For this review, take the finished solid that the model builds, in its own axes (mm). Coordinates: 2 decimals unless noted, no trailing zeros. Write each loop counter-clockwise with the first axis right and the second up, starting at its lowest first coordinate (ties: lowest second). Pieces come first, ordered by that corner, then holes.
1) We need section D-D on y = -16.5. Give the number of separate pieces and of enclosed holes in the cut face, then the cut area to 3 significant figures.
2) We need section C-C on z = -9. Write out the cut boundary in (x, y).
3) We need section B-B on z = 36. Write out the cut boundary in (x, y), then the cut area to 3 significant figures.
4) Insertion check: P1, Ø14.5, axis at x = 15, z = -41.11, coming from the +Y side. The pin has a flat end and moves straight along its axis. Give the tip position at first contact, or say it passes through.
5) To check wall thickness, follow line 1 along X through (y, z) = (-7.5, -72.5); line 2 along X through (y, z) = (-2.25, 85); line 3 along X through (y, z) = (-7.75, 78.5). State the ranges of each line that lie inside material, in increasing order.
6) We need section A-A on z = -41.11. Write out the cut boundary in (x, y), then the cut area to 3 significant figures.
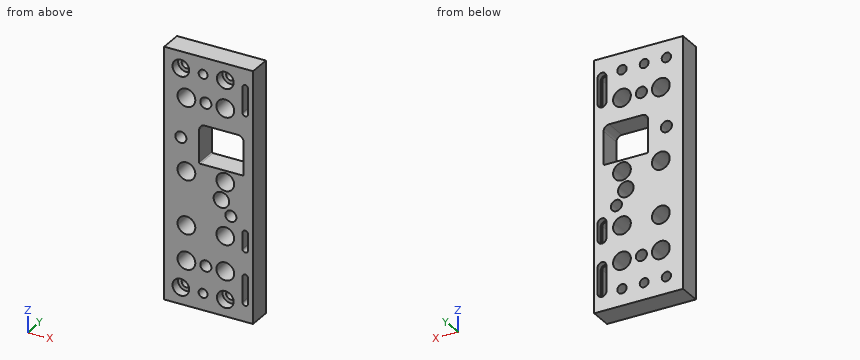
from build123d import *

# Parameters (mm, degrees)
SKETCH1_W                                    = 80
SKETCH1_H                                    = 225
BOSS_EXTRUDE1_DEPTH                          = 20
CUT_EXTRUDE1_REACH                           = 123.063
CUT_EXTRUDE2_REACH                           = 123.063
CUT_EXTRUDE3_DEPTH                           = 5
CBORE_FOR_M8_HEX_SOCKET_HEAD_CAP_SCR_2_COUNT = 2
CBORE_FOR_M8_HEX_SOCKET_HEAD_CAP_SCR_2_PITCH = 40
CBORE_FOR_M8_HEX_SOCKET_HEAD_CAP_SCR_3_COUNT = 2
CBORE_FOR_M8_HEX_SOCKET_HEAD_CAP_SCR_3_PITCH = 199.060292374
CBORE_FOR_M8_HEX_SOCKET_HEAD_CAP_SCR_4_COUNT = 2
CBORE_FOR_M8_HEX_SOCKET_HEAD_CAP_SCR_4_PITCH = 195
F_8_0MM_DOWEL_HOLE1_D                        = 8
F_8_0MM_DOWEL_HOLE1_CSINK_D                  = 8.05
F_8_0MM_DOWEL_HOLE1_CSINK_ANGLE              = 90
CUT_EXTRUDE4_REACH                           = 123.063
SKETCH13_R                                   = 8
CUT_EXTRUDE5_REACH                           = 123.063
SKETCH15_R                                   = 5
CUT_EXTRUDE6_REACH                           = 123.063
SKETCH17_R                                   = 7


with BuildPart() as part:
    # Sketch1 → Boss-Extrude1 (new body)
    with BuildSketch(Plane(origin=(0, 0, 0), x_dir=(1, 0, 0), z_dir=(0, 1, 0))):
        Rectangle(SKETCH1_W, SKETCH1_H)
    extrude(amount=-BOSS_EXTRUDE1_DEPTH)

    # Sketch2 → Cut-Extrude1 (cut, up to next)
    with BuildSketch(Plane(origin=(0, 0, 0), x_dir=(1, 0, 0), z_dir=(0, 1, 0)), mode=Mode.PRIVATE) as cut_extrude1_sk1:
        with BuildLine():
            Line((31.5, -47.14), (31.5, -18.14))
            ThreePointArc((31.5, -18.14), (31.207106781, -17.432893219), (30.5, -17.14))
            Line((30.5, -17.14), (-7.5, -17.14))
            ThreePointArc((-7.5, -17.14), (-8.207106781, -17.432893219), (-8.5, -18.14))
            Line((-8.5, -18.14), (-8.5, -47.14))
            ThreePointArc((-8.5, -47.14), (-7.035533906, -50.675533906), (-3.5, -52.14))
            Line((-3.5, -52.14), (26.5, -52.14))
            ThreePointArc((26.5, -52.14), (30.035533906, -50.675533906), (31.5, -47.14))
        make_face()
    cut_extrude1_tool1 = extrude(cut_extrude1_sk1.sketch, amount=-CUT_EXTRUDE1_REACH, mode=Mode.PRIVATE) & part.part
    add(cut_extrude1_tool1.solids().sort_by_distance((11.5, 0, 34.518764))[0], mode=Mode.SUBTRACT)

    # Sketch3 → Cut-Extrude2 (cut, up to next)
    with BuildSketch(Plane(origin=(0, 0, 0), x_dir=(1, 0, 0), z_dir=(0, 1, 0)), mode=Mode.PRIVATE) as cut_extrude2_sk1:
        with BuildLine():
            Line((35.5, -95.77), (35.5, -72.87))
            ThreePointArc((35.5, -72.87), (33, -70.37), (30.5, -72.87))
            Line((30.5, -72.87), (30.5, -95.77))
            ThreePointArc((30.5, -95.77), (33, -98.27), (35.5, -95.77))
        make_face()
    cut_extrude2_tool1 = extrude(cut_extrude2_sk1.sketch, amount=-CUT_EXTRUDE2_REACH, mode=Mode.PRIVATE) & part.part
    # Sketch3 → Cut-Extrude2 (cut, up to next)
    with BuildSketch(Plane(origin=(0, 0, 0), x_dir=(1, 0, 0), z_dir=(0, 1, 0)), mode=Mode.PRIVATE) as cut_extrude2_sk2:
        with BuildLine():
            Line((35.5, 33.86), (35.5, 48.36))
            ThreePointArc((35.5, 48.36), (33, 50.86), (30.5, 48.36))
            Line((30.5, 48.36), (30.5, 33.86))
            ThreePointArc((30.5, 33.86), (33, 31.36), (35.5, 33.86))
        make_face()
    cut_extrude2_tool2 = extrude(cut_extrude2_sk2.sketch, amount=-CUT_EXTRUDE2_REACH, mode=Mode.PRIVATE) & part.part
    # Sketch3 → Cut-Extrude2 (cut, up to next)
    with BuildSketch(Plane(origin=(0, 0, 0), x_dir=(1, 0, 0), z_dir=(0, 1, 0)), mode=Mode.PRIVATE) as cut_extrude2_sk3:
        with BuildLine():
            Line((35.5, 72.87), (35.5, 95.77))
            ThreePointArc((35.5, 95.77), (33, 98.27), (30.5, 95.77))
            Line((30.5, 95.77), (30.5, 72.87))
            ThreePointArc((30.5, 72.87), (33, 70.37), (35.5, 72.87))
        make_face()
    cut_extrude2_tool3 = extrude(cut_extrude2_sk3.sketch, amount=-CUT_EXTRUDE2_REACH, mode=Mode.PRIVATE) & part.part
    add(cut_extrude2_tool1.solids().sort_by_distance((33, 0, 84.32))[0], mode=Mode.SUBTRACT)
    add(cut_extrude2_tool2.solids().sort_by_distance((33, 0, -41.11))[0], mode=Mode.SUBTRACT)
    add(cut_extrude2_tool3.solids().sort_by_distance((33, 0, -84.32))[0], mode=Mode.SUBTRACT)

    # Sketch4 → Cut-Extrude3 (cut)
    with BuildSketch(Plane(origin=(0, 0, 0), x_dir=(1, 0, 0), z_dir=(0, 1, 0))):
        with BuildLine():
            Line((37, 72.87), (37, 95.77))
            ThreePointArc((37, 95.77), (33, 99.77), (29, 95.77))
            Line((29, 95.77), (29, 72.87))
            ThreePointArc((29, 72.87), (33, 68.87), (37, 72.87))
        make_face()
        with BuildLine():
            Line((37, 33.86), (37, 48.36))
            ThreePointArc((37, 48.36), (33, 52.36), (29, 48.36))
            Line((29, 48.36), (29, 33.86))
            ThreePointArc((29, 33.86), (33, 29.86), (37, 33.86))
        make_face()
        with BuildLine():
            Line((37, -95.77), (37, -72.87))
            ThreePointArc((37, -72.87), (33, -68.87), (29, -72.87))
            Line((29, -72.87), (29, -95.77))
            ThreePointArc((29, -95.77), (33, -99.77), (37, -95.77))
        make_face()
    extrude(amount=-CUT_EXTRUDE3_DEPTH, mode=Mode.SUBTRACT)

    # Sketch8 → CBORE for M8 Hex Socket Head Cap Screw1 (revolve, cut)
    with BuildSketch(Plane(origin=(-25, -20, -97.5), x_dir=(0, 0, -1), z_dir=(1, 0, 0))):
        Polygon((0, 0), (0, 20), (4.2, 20), (4.2, 8.6), (7.5, 8.6), (7.5, 0.025), (7.525, 0), align=None)
    cbore_for_m8_hex_socket_head_cap_screw1 = revolve(axis=Axis((-25, -26.35, -97.5), (0, 1, 0)), mode=Mode.SUBTRACT)

    # CBORE for M8 Hex Socket Head Cap Scr 2: CBORE for M8 Hex Socket Head Cap Screw1 ×2
    with Locations(*[(i * CBORE_FOR_M8_HEX_SOCKET_HEAD_CAP_SCR_2_PITCH, 0, 0) for i in range(1, CBORE_FOR_M8_HEX_SOCKET_HEAD_CAP_SCR_2_COUNT)]):
        add(cbore_for_m8_hex_socket_head_cap_screw1, mode=Mode.SUBTRACT)

    # CBORE for M8 Hex Socket Head Cap Scr 3: CBORE for M8 Hex Socket Head Cap Screw1 ×2
    with Locations(*[Vector(0.2009441437213313, 0, 0.9796027006414901) * (i * CBORE_FOR_M8_HEX_SOCKET_HEAD_CAP_SCR_3_PITCH) for i in range(1, CBORE_FOR_M8_HEX_SOCKET_HEAD_CAP_SCR_3_COUNT)]):
        add(cbore_for_m8_hex_socket_head_cap_screw1, mode=Mode.SUBTRACT)

    # CBORE for M8 Hex Socket Head Cap Scr 4: CBORE for M8 Hex Socket Head Cap Screw1 ×2
    with Locations(*[(0, 0, i * CBORE_FOR_M8_HEX_SOCKET_HEAD_CAP_SCR_4_PITCH) for i in range(1, CBORE_FOR_M8_HEX_SOCKET_HEAD_CAP_SCR_4_COUNT)]):
        add(cbore_for_m8_hex_socket_head_cap_screw1, mode=Mode.SUBTRACT)

    # Ø8.0mm Dowel Hole1 (through all)
    with Locations(Plane(origin=(0, -20, 0), x_dir=(-1, 0, 0), z_dir=(0, -1, 0))):
        with Locations((5, -97.5), (5, 97.5)):
            CounterSinkHole(F_8_0MM_DOWEL_HOLE1_D / 2, F_8_0MM_DOWEL_HOLE1_CSINK_D / 2, counter_sink_angle=F_8_0MM_DOWEL_HOLE1_CSINK_ANGLE)

    # Sketch13 → Cut-Extrude4 (cut, up to next)
    with BuildSketch(Plane(origin=(0, 0, 0), x_dir=(1, 0, 0), z_dir=(0, 1, 0)), mode=Mode.PRIVATE) as cut_extrude4_sk1:
        with Locations(Location((15, 41.11, 0), (0, 0, 270))):
            Circle(SKETCH13_R)
    cut_extrude4_tool1 = extrude(cut_extrude4_sk1.sketch, amount=-CUT_EXTRUDE4_REACH, mode=Mode.PRIVATE) & part.part
    # Sketch13 → Cut-Extrude4 (cut, up to next)
    with BuildSketch(Plane(origin=(0, 0, 0), x_dir=(1, 0, 0), z_dir=(0, 1, 0)), mode=Mode.PRIVATE) as cut_extrude4_sk2:
        with Locations(Location((15, -7, 0), (0, 0, 270))):
            Circle(SKETCH13_R)
    cut_extrude4_tool2 = extrude(cut_extrude4_sk2.sketch, amount=-CUT_EXTRUDE4_REACH, mode=Mode.PRIVATE) & part.part
    # Sketch13 → Cut-Extrude4 (cut, up to next)
    with BuildSketch(Plane(origin=(0, 0, 0), x_dir=(1, 0, 0), z_dir=(0, 1, 0)), mode=Mode.PRIVATE) as cut_extrude4_sk3:
        with Locations(Location((15, -72.5, 0), (0, 0, 270))):
            Circle(SKETCH13_R)
    cut_extrude4_tool3 = extrude(cut_extrude4_sk3.sketch, amount=-CUT_EXTRUDE4_REACH, mode=Mode.PRIVATE) & part.part
    # Sketch13 → Cut-Extrude4 (cut, up to next)
    with BuildSketch(Plane(origin=(0, 0, 0), x_dir=(1, 0, 0), z_dir=(0, 1, 0)), mode=Mode.PRIVATE) as cut_extrude4_sk4:
        with Locations(Location((-20, -72.5, 0), (0, 0, 270))):
            Circle(SKETCH13_R)
    cut_extrude4_tool4 = extrude(cut_extrude4_sk4.sketch, amount=-CUT_EXTRUDE4_REACH, mode=Mode.PRIVATE) & part.part
    # Sketch13 → Cut-Extrude4 (cut, up to next)
    with BuildSketch(Plane(origin=(0, 0, 0), x_dir=(1, 0, 0), z_dir=(0, 1, 0)), mode=Mode.PRIVATE) as cut_extrude4_sk5:
        with Locations(Location((-20, -7, 0), (0, 0, 270))):
            Circle(SKETCH13_R)
    cut_extrude4_tool5 = extrude(cut_extrude4_sk5.sketch, amount=-CUT_EXTRUDE4_REACH, mode=Mode.PRIVATE) & part.part
    # Sketch13 → Cut-Extrude4 (cut, up to next)
    with BuildSketch(Plane(origin=(0, 0, 0), x_dir=(1, 0, 0), z_dir=(0, 1, 0)), mode=Mode.PRIVATE) as cut_extrude4_sk6:
        with Locations(Location((-20, 41.11, 0), (0, 0, 270))):
            Circle(SKETCH13_R)
    cut_extrude4_tool6 = extrude(cut_extrude4_sk6.sketch, amount=-CUT_EXTRUDE4_REACH, mode=Mode.PRIVATE) & part.part
    # Sketch13 → Cut-Extrude4 (cut, up to next)
    with BuildSketch(Plane(origin=(0, 0, 0), x_dir=(1, 0, 0), z_dir=(0, 1, 0)), mode=Mode.PRIVATE) as cut_extrude4_sk7:
        with Locations(Location((-20, 72.5, 0), (0, 0, 270))):
            Circle(SKETCH13_R)
    cut_extrude4_tool7 = extrude(cut_extrude4_sk7.sketch, amount=-CUT_EXTRUDE4_REACH, mode=Mode.PRIVATE) & part.part
    # Sketch13 → Cut-Extrude4 (cut, up to next)
    with BuildSketch(Plane(origin=(0, 0, 0), x_dir=(1, 0, 0), z_dir=(0, 1, 0)), mode=Mode.PRIVATE) as cut_extrude4_sk8:
        with Locations(Location((15, 72.5, 0), (0, 0, 270))):
            Circle(SKETCH13_R)
    cut_extrude4_tool8 = extrude(cut_extrude4_sk8.sketch, amount=-CUT_EXTRUDE4_REACH, mode=Mode.PRIVATE) & part.part
    add(cut_extrude4_tool1.solids().sort_by_distance((15, 0, -41.11))[0], mode=Mode.SUBTRACT)
    add(cut_extrude4_tool2.solids().sort_by_distance((15, 0, 7))[0], mode=Mode.SUBTRACT)
    add(cut_extrude4_tool3.solids().sort_by_distance((15, 0, 72.5))[0], mode=Mode.SUBTRACT)
    add(cut_extrude4_tool4.solids().sort_by_distance((-20, 0, 72.5))[0], mode=Mode.SUBTRACT)
    add(cut_extrude4_tool5.solids().sort_by_distance((-20, 0, 7))[0], mode=Mode.SUBTRACT)
    add(cut_extrude4_tool6.solids().sort_by_distance((-20, 0, -41.11))[0], mode=Mode.SUBTRACT)
    add(cut_extrude4_tool7.solids().sort_by_distance((-20, 0, -72.5))[0], mode=Mode.SUBTRACT)
    add(cut_extrude4_tool8.solids().sort_by_distance((15, 0, -72.5))[0], mode=Mode.SUBTRACT)

    # Sketch15 → Cut-Extrude5 (cut, up to next)
    with BuildSketch(Plane(origin=(0, 0, 0), x_dir=(1, 0, 0), z_dir=(0, 1, 0)), mode=Mode.PRIVATE) as cut_extrude5_sk1:
        with Locations(Location((-2.5, -72.5, 0), (0, 0, 270))):
            Circle(SKETCH15_R)
    cut_extrude5_tool1 = extrude(cut_extrude5_sk1.sketch, amount=-CUT_EXTRUDE5_REACH, mode=Mode.PRIVATE) & part.part
    # Sketch15 → Cut-Extrude5 (cut, up to next)
    with BuildSketch(Plane(origin=(0, 0, 0), x_dir=(1, 0, 0), z_dir=(0, 1, 0)), mode=Mode.PRIVATE) as cut_extrude5_sk2:
        with Locations(Location((-25, -36, 0), (0, 0, 270))):
            Circle(SKETCH15_R)
    cut_extrude5_tool2 = extrude(cut_extrude5_sk2.sketch, amount=-CUT_EXTRUDE5_REACH, mode=Mode.PRIVATE) & part.part
    # Sketch15 → Cut-Extrude5 (cut, up to next)
    with BuildSketch(Plane(origin=(0, 0, 0), x_dir=(1, 0, 0), z_dir=(0, 1, 0)), mode=Mode.PRIVATE) as cut_extrude5_sk3:
        with Locations(Location((20, 22, 0), (0, 0, 270))):
            Circle(SKETCH15_R)
    cut_extrude5_tool3 = extrude(cut_extrude5_sk3.sketch, amount=-CUT_EXTRUDE5_REACH, mode=Mode.PRIVATE) & part.part
    # Sketch15 → Cut-Extrude5 (cut, up to next)
    with BuildSketch(Plane(origin=(0, 0, 0), x_dir=(1, 0, 0), z_dir=(0, 1, 0)), mode=Mode.PRIVATE) as cut_extrude5_sk4:
        with Locations(Location((-2.5, 72.5, 0), (0, 0, 270))):
            Circle(SKETCH15_R)
    cut_extrude5_tool4 = extrude(cut_extrude5_sk4.sketch, amount=-CUT_EXTRUDE5_REACH, mode=Mode.PRIVATE) & part.part
    add(cut_extrude5_tool1.solids().sort_by_distance((-2.5, 0, 72.5))[0], mode=Mode.SUBTRACT)
    add(cut_extrude5_tool2.solids().sort_by_distance((-25, 0, 36))[0], mode=Mode.SUBTRACT)
    add(cut_extrude5_tool3.solids().sort_by_distance((20, 0, -22))[0], mode=Mode.SUBTRACT)
    add(cut_extrude5_tool4.solids().sort_by_distance((-2.5, 0, -72.5))[0], mode=Mode.SUBTRACT)

    # Sketch17 → Cut-Extrude6 (cut, up to next)
    with BuildSketch(Plane(origin=(0, 0, 0), x_dir=(1, 0, 0), z_dir=(0, 1, 0)), mode=Mode.PRIVATE) as cut_extrude6_sk1:
        with Locations(Location((11.5, 9.86, 0), (0, 0, 270))):
            Circle(SKETCH17_R)
    cut_extrude6_tool1 = extrude(cut_extrude6_sk1.sketch, amount=-CUT_EXTRUDE6_REACH, mode=Mode.PRIVATE) & part.part
    add(cut_extrude6_tool1.solids().sort_by_distance((11.5, 0, -9.86))[0], mode=Mode.SUBTRACT)


solid = part.part
Result:
1. separate pieces: 1
1. enclosed holes: 23
1. area: 13,400 mm2
2. outline: (-40, -20) - (4.55, -20) - (4.55, 0) - (-40, 0) - close; (18.45, -20) - (40, -20) - (40, 0) - (18.45, 0) - close
3. outline: (-40, -20) - (-30, -20) - (-30, 0) - (-40, 0) - close; (-20, -20) - (-8.5, -20) - (-8.5, 0) - (-20, 0) - close; (31.5, -20) - (40, -20) - (40, 0) - (31.5, 0) - close
3. area: 600 mm2
4. P1: passes through
5. line 1: x = -40 to -28, -12 to -7.5, 2.5 to 7, 23 to 30.53, 35.47 to 40
5. line 2: x = -40 to 29, 37 to 40
5. line 3: x = -40 to -25.29, -14.71 to 9.71, 20.29 to 30.5, 35.5 to 40
6. outline: (-40, -20) - (-28, -20) - (-28, 0) - (-40, 0) - close; (-12, -20) - (7, -20) - (7, 0) - (-12, 0) - close; (23, -20) - (30.5, -20) - (30.5, -5) - (29, -5) - (29, 0) - (23, 0) - close; (35.5, -20) - (40, -20) - (40, 0) - (37, 0) - (37, -5) - (35.5, -5) - close
6. area: 845 mm2
